Could you check a few things on this model? Use its own coordinates, in mm. Face numbers are marked on the shaded views. A direction names the side the tool comes from. Give positions to 0.01 mm unless a question says otherwise; leave off trailing zeros. Order: outer loops, then holes, each group sorted by start corner. A loop starts at its lowest first (then second) coordinate and runs counter-clockwise, first axis right, second up.
(1) On a 3-axis mill with a long thin cutter (end or side, diameter ignored), from which of +Z, -Z, +X, -X, +Y, -Y can I reach the whole of each face in a straight line? I mean the marked faces 5, 6, 7, 8 and 9. Say none if no direction works.
(2) Imagine slicing it at D-D, the plane z = 2.5. Write out the boundary of the cut face in (x, y).
(3) Imagine slicing it at B-B, the plane x = -148. Write out the boundary of the cut face in (y, z), then the cut area to 3 significant figures.
(4) If we mould it in two halves opening along Y, with no side actions, what happens to the marked faces 1, 2, 3 and 4? For each: released by +Y, released by -Y, zero draft, split by the parting line, or undercut.
(5) Imagine slicing it at A-A, the plane z = 4.7. Write out the boundary of the cut face in (x, y), then the cut area to 3 significant figures.
(6) Imagine slicing it at C-C, the plane y = -146.25. Write out the boundary of the cut face in (x, z).
(7) If I drill on probe 1 along Y at (x, z) = (-148, 3.6); probe 2 along Z at (x, y) = (-138, -138.75); probe 3 along X at (y, z) = (-144, 3), over which ranges is the centre line in solid material (lowest first)?
(8) Will these pins go through, and if not, where does the flat tip stop? pin 1 (2 mm diameter, centred on x = -134, z = 4.5, fed in from -Y); pin 2 (2 mm diameter, centred on x = -160.5, z = 5, fed in from -Y); pin 3 (0.6 mm diameter, centred on x = -134.5, z = 3, fed in from -Y).
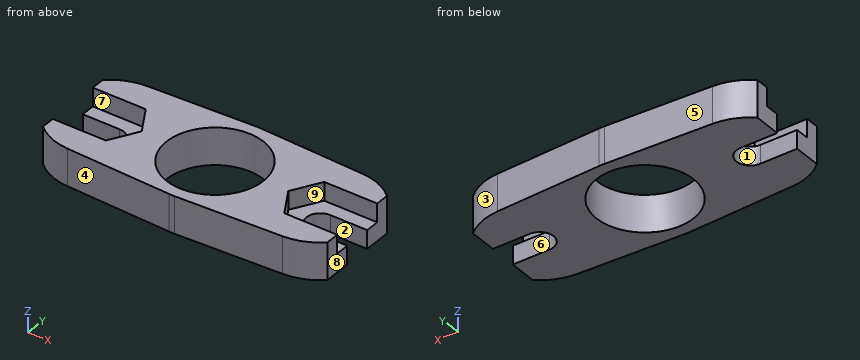
from build123d import *

# Parameters (mm, degrees)
EXTRUDE_1_DEPTH     = 6
SKETCH_2_R          = 5.25
CUT_EXTRUDE_1_DEPTH = 10
CUT_EXTRUDE_2_DEPTH = 2
SKETCH_4_W          = 2
SKETCH_4_H          = 14.987490134
CUT_EXTRUDE_3_DEPTH = 31.8


with BuildPart() as part:
    # Эскиз1 → Бобышка-Вытянуть1 (new body)
    with BuildSketch(Plane.XY):
        with BuildLine():
            Line((-136.336842105, -147.494226215), (-147.714912281, -147.993745067))
            ThreePointArc((-147.714912281, -147.993745067), (-148, -148), (-148.285087719, -147.993745067))
            Line((-148.285087719, -147.993745067), (-159.663157895, -147.494226215))
            ThreePointArc((-159.663157895, -147.494226215), (-161.66336442, -147.05672399), (-163.4, -145.972135955))
            Line((-163.4, -145.972135955), (-163.4, -143))
            Line((-163.4, -143), (-159.4, -143))
            ThreePointArc((-159.4, -143), (-157.9, -141.5), (-159.4, -140))
            Line((-159.4, -140), (-163.4, -140))
            Line((-163.4, -140), (-163.4, -137.027864045))
            ThreePointArc((-163.4, -137.027864045), (-161.66336442, -135.94327601), (-159.663157895, -135.505773785))
            Line((-159.663157895, -135.505773785), (-148.285087719, -135.006254933))
            ThreePointArc((-148.285087719, -135.006254933), (-148, -135), (-147.714912281, -135.006254933))
            Line((-147.714912281, -135.006254933), (-136.336842105, -135.505773785))
            ThreePointArc((-136.336842105, -135.505773785), (-134.33663558, -135.94327601), (-132.6, -137.027864045))
            Line((-132.6, -137.027864045), (-132.6, -140))
            Line((-132.6, -140), (-136.6, -140))
            ThreePointArc((-136.6, -140), (-138.1, -141.5), (-136.6, -143))
            Line((-136.6, -143), (-132.6, -143))
            Line((-132.6, -143), (-132.6, -145.972135955))
            ThreePointArc((-132.6, -145.972135955), (-134.33663558, -147.05672399), (-136.336842105, -147.494226215))
        make_face()
    extrude(amount=EXTRUDE_1_DEPTH)

    # Эскиз2 → Вырез-Вытянуть1 (cut)
    with BuildSketch(Plane.XY.offset(6)):
        with Locations((-148, -141.5)):
            Circle(SKETCH_2_R)
    extrude(amount=-CUT_EXTRUDE_1_DEPTH, mode=Mode.SUBTRACT)

    # Эскиз3 → Вырез-Вытянуть2 (cut)
    with BuildSketch(Plane.XY.offset(6)):
        Polygon((-132.6, -138.5), (-134.867949192, -138.5), (-134.001923789, -140), (-132.6, -140), align=None)
        with BuildLine():
            Line((-134.001923789, -140), (-134.867949192, -138.5))
            Line((-134.867949192, -138.5), (-138.332050808, -138.5))
            Line((-138.332050808, -138.5), (-140.064101615, -141.5))
            Line((-140.064101615, -141.5), (-138.332050808, -144.5))
            Line((-138.332050808, -144.5), (-134.867949192, -144.5))
            Line((-134.867949192, -144.5), (-134.001923789, -143))
            Line((-134.001923789, -143), (-136.6, -143))
            ThreePointArc((-136.6, -143), (-138.1, -141.5), (-136.6, -140))
            Line((-136.6, -140), (-134.001923789, -140))
        make_face()
        Polygon((-132.6, -143), (-134.001923789, -143), (-134.867949192, -144.5), (-132.6, -144.5), align=None)
        with BuildLine():
            Line((-157.667949192, -138.5), (-161.132050808, -138.5))
            Line((-161.132050808, -138.5), (-161.998076211, -140))
            Line((-161.998076211, -140), (-159.4, -140))
            ThreePointArc((-159.4, -140), (-157.9, -141.5), (-159.4, -143))
            Line((-159.4, -143), (-161.998076211, -143))
            Line((-161.998076211, -143), (-161.132050808, -144.5))
            Line((-161.132050808, -144.5), (-157.667949192, -144.5))
            Line((-157.667949192, -144.5), (-155.935898385, -141.5))
            Line((-155.935898385, -141.5), (-157.667949192, -138.5))
        make_face()
        Polygon((-161.998076211, -140), (-161.132050808, -138.5), (-163.4, -138.5), (-163.4, -140), align=None)
        Polygon((-161.998076211, -143), (-163.4, -143), (-163.4, -144.5), (-161.132050808, -144.5), align=None)
    extrude(amount=-CUT_EXTRUDE_2_DEPTH, mode=Mode.SUBTRACT)

    # Эскиз4 → Вырез-Вытянуть3 (cut, through all)
    with BuildSketch(Plane(origin=(-132.6, 0, 0), x_dir=(0, 0, -1), z_dir=(1, 0, 0))):
        with Locations((-1, -141.5)):
            Rectangle(SKETCH_4_W, SKETCH_4_H)
    extrude(amount=-CUT_EXTRUDE_3_DEPTH, mode=Mode.SUBTRACT)


solid = part.part
Answer block:
1. face 5: +Z, -Z, -X, +Y
1. face 6: +Z, -Z, +X
1. face 7: +Z, -X
1. face 8: +Z, -Z, +X, +Y, -Y
1. face 9: +Z, +X
2. outline: (-163.4, -145.97) arc R6 ccw to (-159.66, -147.49) - (-148.29, -147.99) arc R6.5 ccw to (-147.71, -147.99) - (-136.34, -147.49) arc R6 ccw to (-132.6, -145.97) - (-132.6, -143) - (-136.6, -143) arc R1.5 cw to (-136.6, -140) - (-132.6, -140) - (-132.6, -137.03) arc R6 ccw to (-136.34, -135.51) - (-147.71, -135.01) arc R6.5 ccw to (-148.29, -135.01) - (-159.66, -135.51) arc R6 ccw to (-163.4, -137.03) - (-163.4, -140) - (-159.4, -140) arc R1.5 cw to (-159.4, -143) - (-163.4, -143) - close; hole circle Ø10.5 at (-148, -141.5)
3. outline: (-148, 2) - (-146.75, 2) - (-146.75, 6) - (-148, 6) - close; (-136.25, 2) - (-135, 2) - (-135, 6) - (-136.25, 6) - close
3. area: 10.0 mm2
4. face 1: undercut
4. face 2: undercut
4. face 3: released by +Y
4. face 4: released by -Y
5. outline: (-163.4, -145.97) arc R6 ccw to (-159.66, -147.49) - (-148.29, -147.99) arc R6.5 ccw to (-147.71, -147.99) - (-136.34, -147.49) arc R6 ccw to (-132.6, -145.97) - (-132.6, -144.5) - (-138.33, -144.5) - (-140.06, -141.5) - (-138.33, -138.5) - (-132.6, -138.5) - (-132.6, -137.03) arc R6 ccw to (-136.34, -135.51) - (-147.71, -135.01) arc R6.5 ccw to (-148.29, -135.01) - (-159.66, -135.51) arc R6 ccw to (-163.4, -137.03) - (-163.4, -138.5) - (-157.67, -138.5) - (-155.94, -141.5) - (-157.67, -144.5) - (-163.4, -144.5) - close; hole circle Ø10.5 at (-148, -141.5)
5. area: 208 mm2
6. outline: (-163.07, 2) - (-150.24, 2) - (-150.24, 6) - (-163.07, 6) - close; (-145.76, 2) - (-132.93, 2) - (-132.93, 6) - (-145.76, 6) - close
7. probe 1: y = -148 to -146.75, -136.25 to -135
7. probe 2: z = 2 to 4
7. probe 3: x = -163.4 to -152.62, -143.38 to -132.6
8. pin 1: stops at y = -147.28
8. pin 2: stops at y = -147.5
8. pin 3: stops at y = -147.22
